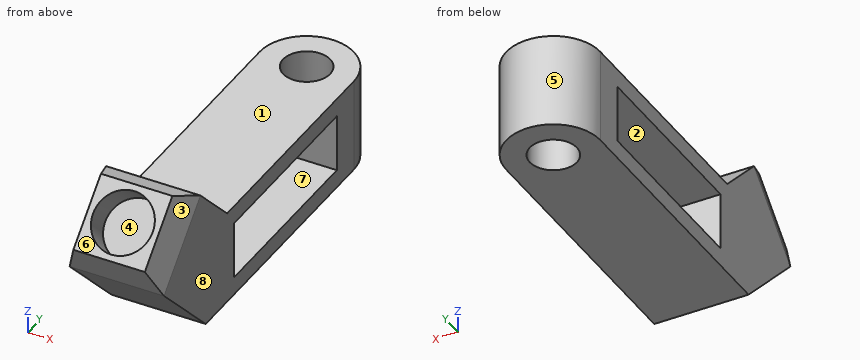
from build123d import *

# Parameters (mm, degrees)
SKETCH11_W          = 38.1
SKETCH11_H          = 38.1
SKETCH12_W          = 38.1
SKETCH12_H          = 38.1
BOSS_EXTRUDE5_DEPTH = 12.7
BOSS_EXTRUDE5_TAPER = 20
BOSS_EXTRUDE6_DEPTH = 38.1
SKETCH14_R          = 9.525
CUT_EXTRUDE2_DEPTH  = 38.1
SKETCH15_R          = 12.065
CUT_EXTRUDE3_DEPTH  = 12.7
SKETCH16_W          = 23.310601064
SKETCH16_H          = 76.2
CUT_EXTRUDE4_DEPTH  = 59.830675793


with BuildPart() as part:
    # Sweep1: sweep along a path in Sketch10
    with BuildLine(Plane(origin=(0, 0, 0), x_dir=(0, 0, -1), z_dir=(1, 0, 0))) as sweep1_path:
        Line((0, 96.393), (0, -5.207))
        Line((0, -5.207), (-25.324322261, -30.531322261))
    # Sketch11 → Sweep1 (sweep)
    with BuildSketch(Plane(origin=(0, 96.393, 0), x_dir=(1, 0, 0), z_dir=(0, 1, 0))):
        Rectangle(SKETCH11_W, SKETCH11_H)
    sweep(path=sweep1_path.line, transition=Transition.RIGHT)

    # Sketch12 → Boss-Extrude5 (add)
    with BuildSketch(Plane(origin=(0, -27.927822261, 27.927822261), x_dir=(1, 0, 0), z_dir=(0, -0.7071067811865461, 0.7071067811865489))):
        with Locations((0, -3.68190501)):
            Rectangle(SKETCH12_W, SKETCH12_H)
    extrude(amount=BOSS_EXTRUDE5_DEPTH, taper=BOSS_EXTRUDE5_TAPER)

    # Sketch13 → Boss-Extrude6 (add)
    with BuildSketch(Plane(origin=(0, 0, -19.05), x_dir=(-1, 0, 0), z_dir=(0, 0, -1))):
        with BuildLine():
            Line((-19.05, 96.393), (19.05, 96.393))
            ThreePointArc((19.05, 96.393), (0, 115.443), (-19.05, 96.393))
        make_face()
    extrude(amount=-BOSS_EXTRUDE6_DEPTH)

    # Sketch14 → Cut-Extrude2 (cut)
    with BuildSketch(Plane.XY.offset(19.05)):
        with Locations((0, 96.393)):
            Circle(SKETCH14_R)
    extrude(amount=-CUT_EXTRUDE2_DEPTH, mode=Mode.SUBTRACT)

    # Sketch15 → Cut-Extrude3 (cut)
    with BuildSketch(Plane(origin=(0, -36.908078382, 36.908078382), x_dir=(1, 0, 0), z_dir=(0, -0.7071067811865461, 0.7071067811865489))):
        with Locations(Location((0, -3.68190501, 0), (0, 0, 270))):
            Circle(SKETCH15_R)
    extrude(amount=-CUT_EXTRUDE3_DEPTH, mode=Mode.SUBTRACT)

    # Sketch16 → Cut-Extrude4 (cut)
    with BuildSketch(Plane(origin=(19.05, 0, 0), x_dir=(0, 0, -1), z_dir=(1, 0, 0))):
        with Locations((0, 45.72)):
            Rectangle(SKETCH16_W, SKETCH16_H)
    extrude(amount=-CUT_EXTRUDE4_DEPTH, mode=Mode.SUBTRACT)


solid = part.part
Part model, mm, in its own coordinate system. Face numbers are marked on the shaded views. A direction names the side the tool comes from. Give positions to 0.01 mm unless a question says otherwise; leave off trailing zeros. Order: outer loops, then holes, each group sorted by start corner. A loop starts at its lowest first (then second) coordinate and runs counter-clockwise, first axis right, second up. Notation, with made-up numbers: (32, -17.75) -> (47, -17.75) arc R33 cw to (47, 16.25) -> close; hole circle Ø2 at (15.5, -15). An arc over 180 degrees is marked (long way). Use one line per item in the form item = value.
(1) Saw through at C-C (x = 2). Write the cut outline in (y, z).
Solution:
outline = (-49.71, 24.1) -> (-44, 11.85) -> (-13.1, -19.05) -> (87.08, -19.05) -> (87.08, 19.05) -> (2.68, 19.05) -> (-17.06, 38.79) -> (-29.31, 44.51) -> (-31.1, 42.72) -> (-22.12, 33.74) -> (-38.94, 16.91) -> (-47.92, 25.89) -> close; (105.71, -19.05) -> (115.34, -19.05) -> (115.34, 19.05) -> (105.71, 19.05) -> close; hole (7.62, -11.66) -> (83.82, -11.66) -> (83.82, 11.66) -> (7.62, 11.66) -> close
(2) Saw through at D-D (x = -16). Write the cut outline in (y, z), then the cut area to 3 significant figures.
Solution:
outline = (-47.77, 19.94) -> (-44, 11.85) -> (-13.1, -19.05) -> (106.73, -19.05) -> (106.73, 19.05) -> (2.68, 19.05) -> (-17.06, 38.79) -> (-25.14, 42.56) -> close; hole (7.62, -11.66) -> (83.82, -11.66) -> (83.82, 11.66) -> (7.62, 11.66) -> close
area = 4,150 mm²
(3) Pull direction Y, two halves, no side cores. Call the marked faces 5, 6, 7 and 8: +Y half, -Y half, draft (parallel to the pull), parting line (faces both ways), or undercut.
Solution:
face_5 = +Y half
face_6 = -Y half
face_7 = undercut
face_8 = draft
(4) Tool access for the marked faces 1, 2, 3 and 4: list every direction of +Z, -Z, +X, -X, +Y, -Y with a clear straight run to the whole face (end or side of a thin tool).
Solution:
face_1 = +Z, +X, -X, +Y
face_2 = +X, -X
face_3 = +Z, +X, -Y
face_4 = none
(5) Saw through at A-A (y = 55). Write the cut outline in (x, z), then the cut area to 3 significant figures.
Solution:
outline = (-19.05, -19.05) -> (19.05, -19.05) -> (19.05, -11.66) -> (-19.05, -11.66) -> close; (-19.05, 11.66) -> (19.05, 11.66) -> (19.05, 19.05) -> (-19.05, 19.05) -> close
area = 563 mm²
(6) Saw through at B-B (z = -7). Write the cut outline in (x, y) (3 decimals).
Solution:
outline = (-19.05, -25.148) -> (19.05, -25.148) -> (19.05, 7.62) -> (-19.05, 7.62) -> close; (-19.05, 83.82) -> (19.05, 83.82) -> (19.05, 96.393) arc R19.05 ccw to (-19.05, 96.393) -> close; hole circle Ø19.05 at (0, 96.393)
(7) Flat gauge pins, fed straight in: P1, Ø1.5, axis at x = 9.5, y = -20, coming from the -Z side; P2, Ø6, axis at x = 1, y = 73.5, coming from the +Z side; P3, Ø7, axis at x = 9, z = 1, coming from the -Y side. Where does each tip first touch, or does it go through?
Solution:
P1 = -12.9
P2 = 19.05
P3 = -36.65
(8) Drill centre lines: line 1 (Z direction, x = 3.5, y = 42); line 2 (Y direction, x = 0, z = -7); line 3 (Y direction, x = 0, z = -2). Where is each one in solid material? Low to high. Write a range as from..to.
Solution:
line_1 = -19.05..-11.66, 11.66..19.05
line_2 = -25.15..7.62, 83.82..86.87, 105.92..115.44
line_3 = -30.15..7.62, 83.82..86.87, 105.92..115.44
